from build123d import *

# Parameters (mm, degrees)
F1_DEPTH = 4
F0_W     = 7
F0_H     = 7
F2_DEPTH = 10
F3_SIZE  = 5.99999
F4_R     = 1.5


# Not quite as in the source:
# - a fillet or chamfer is up to 0.001 mm smaller than in the source, because OpenCascade refuses the exact size


with BuildPart() as f1:
    # F0 (on Top) → F1 (new body)
    with BuildSketch(Plane.XY):
        Polygon((43.5, 25), (-43.5, 25), (-43.5, 18), (-50.5, 18), (-50.5, -18), (-43.5, -18), (-43.5, -25), (43.5, -25), (43.5, -18), (50.5, -18), (50.5, 18), (43.5, 18), align=None)
    extrude(amount=F1_DEPTH)

    # F0 (on Top) → F2 (join)
    with BuildSketch(Plane.XY):
        with Locations((-47, 21.5)):
            Rectangle(F0_W, F0_H)
        with Locations((-47, -21.5)):
            Rectangle(F0_W, F0_H)
        with Locations((47, 21.5)):
            Rectangle(F0_W, F0_H)
        with Locations((47, -21.5)):
            Rectangle(F0_W, F0_H)
    extrude(amount=F2_DEPTH)

    # F3 (size 6 in the source; OpenCascade refuses exactly that, so slightly less here)
    f3_edges = [f1.edges().sort_by_distance(p)[0] for p in [
        (-43.5, 18, 7),
        (-47, 18, 10),
        (-43.5, 21.5, 10),
        (43.5, 21.5, 10),
        (47, 18, 10),
        (47, -18, 10),
        (43.5, -21.5, 10),
        (-43.5, -21.5, 10),
        (-47, -18, 10),
    ]]
    chamfer(f3_edges, length=F3_SIZE)

    # F4
    f4_edges = [f1.edges().sort_by_distance(p)[0] for p in [
        (-50.5, 0, 0),
        (0, -25, 0),
        (50.5, 0, 0),
        (0, 25, 0),
    ]]
    fillet(f4_edges, radius=F4_R)


solid = f1.part
Input: part model. Units: mm. Frame: model coordinates. A direction names the side the tool comes from. Give positions to 0.01 mm unless a question says otherwise; leave off trailing zeros. Write each loop counter-clockwise with the first axis right and the second up, starting at its lowest first coordinate (ties: lowest second). Pieces come first, ordered by that corner, then holes. Notation, with made-up numbers: M 70,-21.75 L 102,-21.75 A16 ccw 102,5.25 Z; hole C 75,54.25 d3. An arc over 180 degrees is marked long. Use one line per item in the form item = value.
1. Cut plane B-B on y = 8.5. Return loops of the section in (x, z), and give its area (3 significant figures).
Outcome:
outline = M -50.5,1.5 A1.5 ccw -49,0 L 49,0 A1.5 ccw 50.5,1.5 L 50.5,4 L -50.5,4 Z
area = 403 mm²
2. Cut plane A-A on z = 6.25. Return loops of the section in (x, y).
Outcome:
outline = M -50.5,-25 L -45.75,-25 L -45.75,-20.25 L -50.5,-20.25 Z; M -50.5,20.25 L -49.5,20.25 L -45.75,24 L -45.75,25 L -50.5,25 Z; M 45.75,-25 L 50.5,-25 L 50.5,-20.25 L 45.75,-20.25 Z; M 45.75,20.25 L 50.5,20.25 L 50.5,25 L 45.75,25 Z
3. Reachability of faces 5 (the face through (45.9, 22.2, 6.4)), 6 (the face through (-47.7, 22.1, 6.3)), 7 (the face through (-50, 21, 7)) from +Z, -Z, +X, -X, +Y, -Y: full face, straight path, thin tool, end or side. Return the list, or none.
Outcome:
face_5 = +Z, +Y, -Y
face_6 = +Z
face_7 = +Z, +X, -X
4. Cut plane C-C on x = -33. Return loops of the section in (y, z).
Outcome:
outline = M -25,1.5 A1.5 ccw -23.5,0 L 23.5,0 A1.5 ccw 25,1.5 L 25,4 L -25,4 Z
5. Ray query, L1, parallel to Z at x = 37, y = 15; L2, parallel to Y at x = -31.5, z = 1.25; L3, parallel to X at y = -0.5, z = 0.75. Return the intervals inside material, ascending.
Outcome:
L1 = 0 to 4
L2 = -24.98 to 24.98
L3 = -50.3 to 50.3
6. First-contact query: P1, Ø6, axis at x = 24.5, z = 1, coming from the +Y side; P2, Ø12, axis at x = -40.5, y = 1, coming from the +Z side. Flat tips, straight axial feed; report the tip coordinate or a pass-through.
Outcome:
P1 = 25
P2 = 4
7. Mould query, pull axis Y, two halves, no side actions, for faces 1 (the face through (-46.5, 24.5, 7)), 2 (the face through (48, -20, 6)), 3 (the face through (-0.2, -25, 3.5)), 4 (the face through (-0.2, 25, 3.5)). Classes: released by +Y, released by -Y, zero draft, split by the parting line, or undercut.
Outcome:
face_1 = zero draft
face_2 = undercut
face_3 = released by -Y
face_4 = released by +Y
